Source: three-view drawing plus pictorial views. Frame: mm from the lowest corner of the part. Give positions to 0.01 mm unless a question says otherwise; leave off trailing zeros. Loops run counter-clockwise (first coordinate to the right, second up) from the corner with the lowest first, then second, coordinate; pieces in that order, holes last. Notation, with made-up numbers: M 6,-30 L 48,-30 A27 ccw 48,-12 Z; hole C 30,3 d11. An arc over 180 degrees is marked long. Answer as a JSON object with one key per item and string values. Group by question number.
1) Section query C-C on x = 8.5. Return loops of the section in (y, z).
2) Section query D-D on y = 21.5. Return loops of the section in (x, z) (1 decimal).
3) Section query A-A on z = 13.5. Return loops of the section in (x, y) (1 decimal), plus the area to 4 significant figures.
4) First-contact query: P1, Ø6, axis at y = 38, z = 2, coming from the -X side (1 decimal); P2, Ø3.5, axis at x = 45.01, y = 3.99, coming from the -Z side. Flat tips, straight axial feed; report the tip coordinate or a pass-through.
5) Ray query, L1, parallel to X at y = 24, z = 12.5 (1 decimal); L2, parallel to Y at x = 5.5, z = 6.5 (1 decimal); L3, parallel to Y at x = 11, z = 2 (1 decimal). Return the intervals inside material, ascending.
6) Draft query along X for the marked faces 1, 2, 3 and 4. Return one class per face: +X half, -X half, draft (parallel to the pull), parting line (faces both ways), or undercut.
7) Section query B-B on y = 43.5. Return loops of the section in (x, z) (1 decimal).
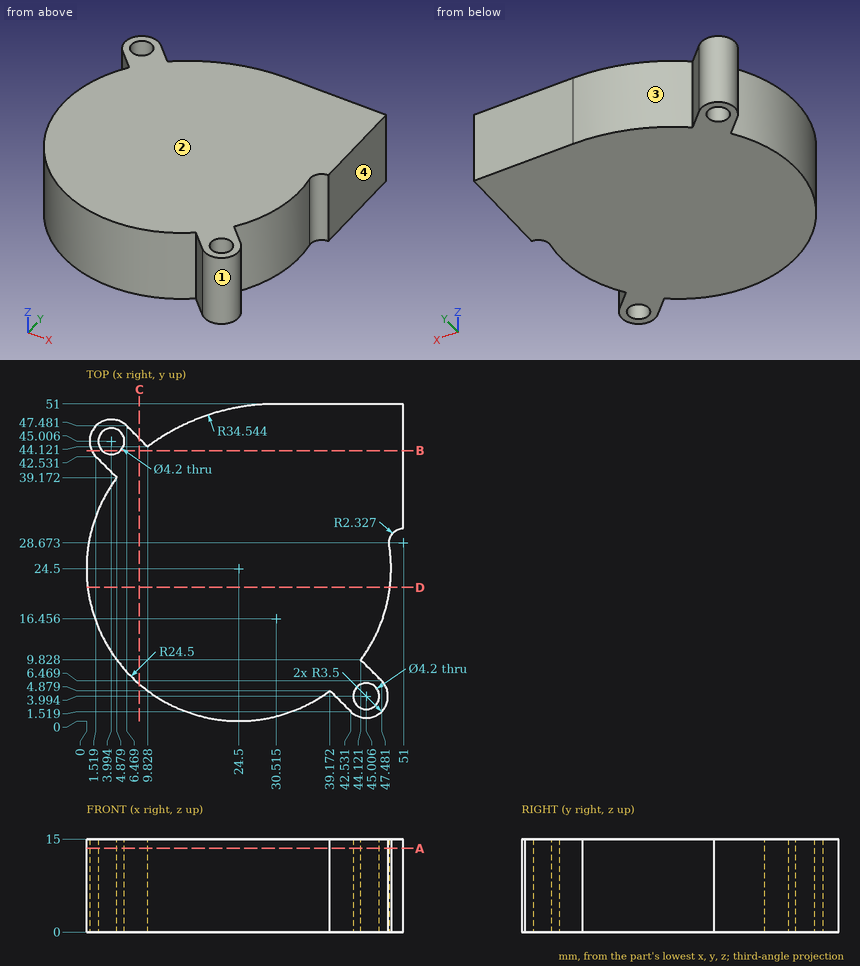
Output:
{
 "1": {"outline": "M 5.95,0 L 45.45,0 L 45.45,15 L 5.95,15 Z"},
 "2": {"outline": "M 0.2,0 L 48.8,0 L 48.8,15 L 0.2,15 Z"},
 "3": {"outline": "M 1.5,42.5 L 4.9,39.2 A24.5 ccw 39.2,4.9 L 42.5,1.5 A3.5 ccw 47.5,6.5 L 44.1,9.8 A24.5 ccw 48.7,28.3 A2.3 cw 51,31 L 51,51 L 30.5,51 A34.5 ccw 9.8,44.1 L 6.5,47.5 A3.5 ccw Z; hole C 4,45 d4.2; hole C 45,4 d4.2", "area": "2,185 mm^2"},
 "4": {"P1": "stops at x = 2.4", "P2": "passes through"},
 "5": {"L1": "x = 0 to 49", "L2": "y = 9 to 43.5, 46.5 to 48.2", "L3": "y = 4.1 to 45"},
 "6": {"face 1": "undercut", "face 2": "draft", "face 3": "undercut", "face 4": "+X half"},
 "7": {"outline": "M 0.8,0 L 2.5,0 L 2.5,15 L 0.8,15 Z; M 5.5,0 L 51,0 L 51,15 L 5.5,15 Z"}
}
